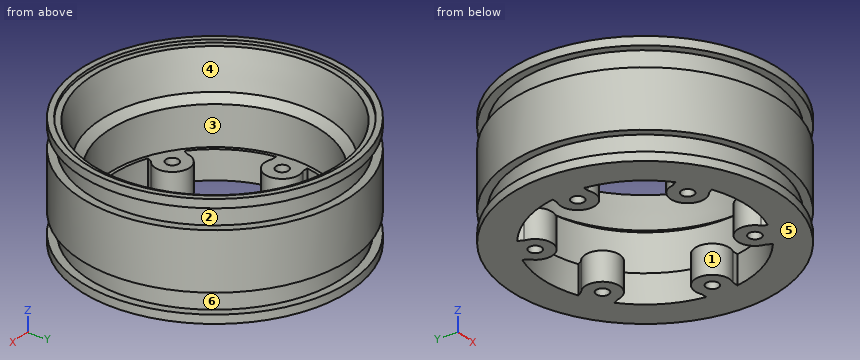
from build123d import *

# Parameters (mm, degrees)
CYLINDER154_R             = 1.1
CYLINDER154_DEPTH         = 5
BOX024_W                  = 2
BOX024_H                  = 5.5
BOX024_DEPTH              = 5
BOX023_W                  = 0.75
BOX023_H                  = 8
BOX023_DEPTH              = 5
CYLINDER153_R             = 3
CYLINDER153_DEPTH         = 5
CUT033013_PLACEMENT_ANGLE = 120
CYLINDER157_R             = 1.1
CYLINDER157_DEPTH         = 5
CUT033016_PLACEMENT_ANGLE = 60
CYLINDER155_R             = 1.1
CYLINDER155_DEPTH         = 5
CUT033014_PLACEMENT_ANGLE = 180
CYLINDER158_R             = 1.1
CYLINDER158_DEPTH         = 5
CYLINDER156_R             = 1.1
CYLINDER156_DEPTH         = 5
CUT033015_PLACEMENT_ANGLE = 240
CYLINDER152_R             = 1.1
CYLINDER152_DEPTH         = 5
CUT033012_PLACEMENT_ANGLE = 60
CYLINDER143_R             = 18.5
CYLINDER143_DEPTH         = 7
CYLINDER144_R             = 22.5
CYLINDER144_DEPTH         = 0.5
CYLINDER145_R             = 20
CYLINDER145_DEPTH         = 7
CYLINDER142_R             = 17.9
CYLINDER142_DEPTH         = 20
CYLINDER138_R             = 22.1
CYLINDER138_DEPTH         = 17
CYLINDER139_R             = 23.5
CYLINDER139_DEPTH         = 17
CYLINDER137_R             = 23.5
CYLINDER137_DEPTH         = 20
CYLINDER140_R             = 22
CYLINDER140_DEPTH         = 17
CYLINDER141_R             = 23.5
CYLINDER141_DEPTH         = 10
CUT033011_PLACEMENT_ANGLE = 180
CHAMFER_SIZE2             = 6.499
CHAMFER_SIZE              = 1.5


with BuildPart() as cylinder154:
    # Cylinder154 → Cylinder154 (new body)
    with BuildSketch(Plane(origin=(15.5, 0, 15), x_dir=(1, 0, 0), z_dir=(0, 0, 1))):
        Circle(CYLINDER154_R)
    extrude(amount=CYLINDER154_DEPTH)


with BuildPart() as cube024:
    # Box024 → Box024 (new body)
    with BuildSketch(Plane(origin=(16.5, -2.75, 15), x_dir=(1, 0, 0), z_dir=(0, 0, 1))):
        with Locations((1, 2.75)):
            Rectangle(BOX024_W, BOX024_H)
    extrude(amount=BOX024_DEPTH)


with BuildPart() as cube023:
    # Box023 → Box023 (new body)
    with BuildSketch(Plane(origin=(18.2, -4, 15), x_dir=(1, 0, 0), z_dir=(0, 0, 1))):
        with Locations((0.375, 4)):
            Rectangle(BOX023_W, BOX023_H)
    extrude(amount=BOX023_DEPTH)


with BuildPart() as cylinder153:
    # Cylinder153 → Cylinder153 (new body)
    with BuildSketch(Plane(origin=(15.5, 0, 15), x_dir=(1, 0, 0), z_dir=(0, 0, 1))):
        Circle(CYLINDER153_R)
    extrude(amount=CYLINDER153_DEPTH)


with BuildPart() as cut033013:
    # Fusion040005 base: copy of Cylinder153
    add(cylinder153.part)

    # Fusion040005: union Cube024, Cube023
    add(cube024.part)
    add(cube023.part)

    # Cut033013: cut Cylinder154
    add(cylinder154.part, mode=Mode.SUBTRACT)


with BuildPart() as cut033013_1:
    # Cut033013 placement: moved
    add(cut033013.part.moved(Location((0, 0, 9))).rotate(Axis((0, 0, 9), (0, 0, 1)), CUT033013_PLACEMENT_ANGLE))


with BuildPart() as cylinder157:
    # Cylinder157 → Cylinder157 (new body)
    with BuildSketch(Plane(origin=(15.5, 0, 15), x_dir=(1, 0, 0), z_dir=(0, 0, 1))):
        Circle(CYLINDER157_R)
    extrude(amount=CYLINDER157_DEPTH)


with BuildPart() as cut033016:
    # Fusion040008 base: copy of Cylinder153
    add(cylinder153.part)

    # Fusion040008: union Cube024, Cube023
    add(cube024.part)
    add(cube023.part)

    # Cut033016: cut Cylinder157
    add(cylinder157.part, mode=Mode.SUBTRACT)


with BuildPart() as cut033016_1:
    # Cut033016 placement: moved
    add(cut033016.part.moved(Location((0, 0, 9))).rotate(Axis((0, 0, 9), (0, 0, -1)), CUT033016_PLACEMENT_ANGLE))


with BuildPart() as cylinder155:
    # Cylinder155 → Cylinder155 (new body)
    with BuildSketch(Plane(origin=(15.5, 0, 15), x_dir=(1, 0, 0), z_dir=(0, 0, 1))):
        Circle(CYLINDER155_R)
    extrude(amount=CYLINDER155_DEPTH)


with BuildPart() as cut033014:
    # Fusion040006 base: copy of Cylinder153
    add(cylinder153.part)

    # Fusion040006: union Cube024, Cube023
    add(cube024.part)
    add(cube023.part)

    # Cut033014: cut Cylinder155
    add(cylinder155.part, mode=Mode.SUBTRACT)


with BuildPart() as cut033014_1:
    # Cut033014 placement: moved
    add(cut033014.part.moved(Location((0, 0, 9))).rotate(Axis((0, 0, 9), (0, 0, 1)), CUT033014_PLACEMENT_ANGLE))


with BuildPart() as cylinder158:
    # Cylinder158 → Cylinder158 (new body)
    with BuildSketch(Plane(origin=(15.5, 0, 15), x_dir=(1, 0, 0), z_dir=(0, 0, 1))):
        Circle(CYLINDER158_R)
    extrude(amount=CYLINDER158_DEPTH)


with BuildPart() as cut033006:
    # Fusion040009 base: copy of Cylinder153
    add(cylinder153.part)

    # Fusion040009: union Cube024, Cube023
    add(cube024.part)
    add(cube023.part)

    # Cut033006: cut Cylinder158
    add(cylinder158.part, mode=Mode.SUBTRACT)


with BuildPart() as cut033006_1:
    # Cut033006 placement: moved
    add(cut033006.part.moved(Location((0, 0, 9))))


with BuildPart() as cylinder156:
    # Cylinder156 → Cylinder156 (new body)
    with BuildSketch(Plane(origin=(15.5, 0, 15), x_dir=(1, 0, 0), z_dir=(0, 0, 1))):
        Circle(CYLINDER156_R)
    extrude(amount=CYLINDER156_DEPTH)


with BuildPart() as cut033015:
    # Fusion040007 base: copy of Cylinder153
    add(cylinder153.part)

    # Fusion040007: union Cube024, Cube023
    add(cube024.part)
    add(cube023.part)

    # Cut033015: cut Cylinder156
    add(cylinder156.part, mode=Mode.SUBTRACT)


with BuildPart() as cut033015_1:
    # Cut033015 placement: moved
    add(cut033015.part.moved(Location((0, 0, 9))).rotate(Axis((0, 0, 9), (0, 0, 1)), CUT033015_PLACEMENT_ANGLE))


with BuildPart() as cylinder152:
    # Cylinder152 → Cylinder152 (new body)
    with BuildSketch(Plane(origin=(15.5, 0, 15), x_dir=(1, 0, 0), z_dir=(0, 0, 1))):
        Circle(CYLINDER152_R)
    extrude(amount=CYLINDER152_DEPTH)


with BuildPart() as fusion040010:
    # Fusion040004 base: copy of Cylinder153
    add(cylinder153.part)

    # Fusion040004: union Cube024, Cube023
    add(cube024.part)
    add(cube023.part)

    # Cut033012: cut Cylinder152
    add(cylinder152.part, mode=Mode.SUBTRACT)


with BuildPart() as fusion040010_1:
    # Cut033012 placement: moved
    add(fusion040010.part.moved(Location((0, 0, 9))).rotate(Axis((0, 0, 9), (0, 0, 1)), CUT033012_PLACEMENT_ANGLE))

    # Fusion040010: union Cut033013, Cut033016, Cut033014, Cut033006, Cut033015
    add(cut033013_1.part)
    add(cut033016_1.part)
    add(cut033014_1.part)
    add(cut033006_1.part)
    add(cut033015_1.part)


with BuildPart() as cylinder143:
    # Cylinder143 → Cylinder143 (new body)
    with BuildSketch(Plane.XY.offset(8)):
        Circle(CYLINDER143_R)
    extrude(amount=CYLINDER143_DEPTH)


with BuildPart() as cone001:
    # Cone001 → Cone001 (revolve)
    with BuildSketch(Plane(origin=(0, 0, 7), x_dir=(1, 0, 0), z_dir=(0, -1, 0))):
        Polygon((0, 0), (20, 0), (12, 6), (0, 6), align=None)
    revolve(axis=Axis((0, 0, 7), (0, 0, 1)))


with BuildPart() as cylinder144:
    # Cylinder144 → Cylinder144 (new body)
    with BuildSketch(Plane.XY):
        Circle(CYLINDER144_R)
    extrude(amount=CYLINDER144_DEPTH)


with BuildPart() as cylinder145:
    # Cylinder145 → Cylinder145 (new body)
    with BuildSketch(Plane.XY):
        Circle(CYLINDER145_R)
    extrude(amount=CYLINDER145_DEPTH)


with BuildPart() as cylinder142:
    # Cylinder142 → Cylinder142 (new body)
    with BuildSketch(Plane.XY):
        Circle(CYLINDER142_R)
    extrude(amount=CYLINDER142_DEPTH)


with BuildPart() as cylinder138:
    # Cylinder138 → Cylinder138 (new body)
    with BuildSketch(Plane.XY):
        Circle(CYLINDER138_R)
    extrude(amount=CYLINDER138_DEPTH)


with BuildPart() as cut033005:
    # Cylinder139 → Cylinder139 (new body)
    with BuildSketch(Plane.XY):
        Circle(CYLINDER139_R)
    extrude(amount=CYLINDER139_DEPTH)

    # Cut033005: cut Cylinder138
    add(cylinder138.part, mode=Mode.SUBTRACT)


with BuildPart() as cut033005_1:
    # Cut033005 placement: moved
    add(cut033005.part.moved(Location((0, 0, 1.5))))


with BuildPart() as cut033004:
    # Cylinder137 → Cylinder137 (new body)
    with BuildSketch(Plane.XY):
        Circle(CYLINDER137_R)
    extrude(amount=CYLINDER137_DEPTH)

    # Cut033004: cut Cut033005
    add(cut033005_1.part, mode=Mode.SUBTRACT)


with BuildPart() as cylinder140:
    # Cylinder140 → Cylinder140 (new body)
    with BuildSketch(Plane.XY):
        Circle(CYLINDER140_R)
    extrude(amount=CYLINDER140_DEPTH)


with BuildPart() as obj1:
    # Cylinder141 → Cylinder141 (new body)
    with BuildSketch(Plane.XY.offset(0.5)):
        Circle(CYLINDER141_R)
    extrude(amount=CYLINDER141_DEPTH)

    # Cut033003: cut Cylinder140
    add(cylinder140.part, mode=Mode.SUBTRACT)


with BuildPart() as obj1_1:
    # Cut033003 placement: moved
    add(obj1.part.moved(Location((0, 0, 4.5))))

    # Fusion040003: union Cut033004
    add(cut033004.part)

    # Cut033007: cut Cylinder142
    add(cylinder142.part, mode=Mode.SUBTRACT)

    # Cut033009: cut Cylinder145
    add(cylinder145.part, mode=Mode.SUBTRACT)

    # Cut033008: cut Cylinder144
    add(cylinder144.part, mode=Mode.SUBTRACT)

    # Cut033010: cut Cone001
    add(cone001.part, mode=Mode.SUBTRACT)

    # Cut033011: cut Cylinder143
    add(cylinder143.part, mode=Mode.SUBTRACT)


with BuildPart() as obj1_2:
    # Cut033011 placement: moved
    add(obj1_1.part.moved(Location((0, 0, 44))).rotate(Axis((0, 0, 44), (0, 1, 0)), CUT033011_PLACEMENT_ANGLE))

    # Fusion040011: union Fusion040010
    add(fusion040010_1.part)


with BuildPart() as obj1_3:
    # Fusion040011 placement: moved
    add(obj1_2.part.moved(Location((0, 0, -44))))

    # Chamfer
    chamfer_edges = [obj1_3.edges().sort_by_distance(p)[0] for p in [
        (20, 0, -0.5),
    ]]
    chamfer_side = obj1_3.faces().sort_by_distance((21.863604, 0, -0.5))[0]
    chamfer(chamfer_edges, length=CHAMFER_SIZE, length2=CHAMFER_SIZE2, reference=chamfer_side)


solid = obj1_3.part
Input: part model. Units: mm. Frame: model coordinates. Face numbers are marked on the shaded views. A direction names the side the tool comes from. Give positions to 0.01 mm unless a question says otherwise; leave off trailing zeros. Order: outer loops, then holes, each group sorted by start corner. A loop starts at its lowest first (then second) coordinate and runs counter-clockwise, first axis right, second up.
Q1. Contact query for flat-ended pins moving along their axis: pin 1 Ø1 at (y, z) = (-1.5, -4) entering from +X; pin 2 Ø3 at (x, y) = (7.75, 13.42) entering from +Z; pin 3 Ø1.5 at (y, z) = (-0.5, -15.5) entering from +X; pin 4 Ø14 at (x, y) = (3.5, 1.5) entering from +Z. Output: stop coordinate, or through.
Checked values:
pin 1: stops at x = 22.08
pin 2: stops at z = -15
pin 3: stops at x = 23.5
pin 4: passes through
Q2. Draft query along X for the marked faces 4, 5 and 6. Return one class per face: +X half, -X half, draft (parallel to the pull), parting line (faces both ways), or undercut.
Checked values:
face 4: undercut
face 5: draft
face 6: parting line
Q3. Section B-B on z = -10. Output: boundary loops of the cut face in (x, y), and give its area (3 significant figures).
Checked values:
outline: circle Ø47 at (0, 0); hole circle Ø37 at (0, 0)
area: 660 mm2
Q4. Section A-A on z = -16.5. State how many separate pieces and enclosed holes the cut face has, and give its area (3 significant figures).
Checked values:
separate pieces: 1
enclosed holes: 7
area: 669 mm2
Q5. Ray query, probe 1 along Z at (x, y) = (-12, -19); probe 2 along Y at (x, z) = (0, -0.2); probe 3 along X at (y, z) = (-8, -14). Return the intervals inside material, ascending.
Checked values:
probe 1: z = -20 to -18.5, -15 to -5, -1.5 to -0.5
probe 2: y = -23.5 to -22.5, 22.5 to 23.5
probe 3: x = -22.1 to -16.68, 16.68 to 22.1
Q6. Set-up query: the marked faces 1, 2 and 3. Return all of +Z, -Z, +X, -X, +Y, -Y with unobstructed straight access to the full face (end or side cutting, diameter ignored); none if empty.
Checked values:
face 1: +Z, -Z
face 2: none
face 3: +Z
